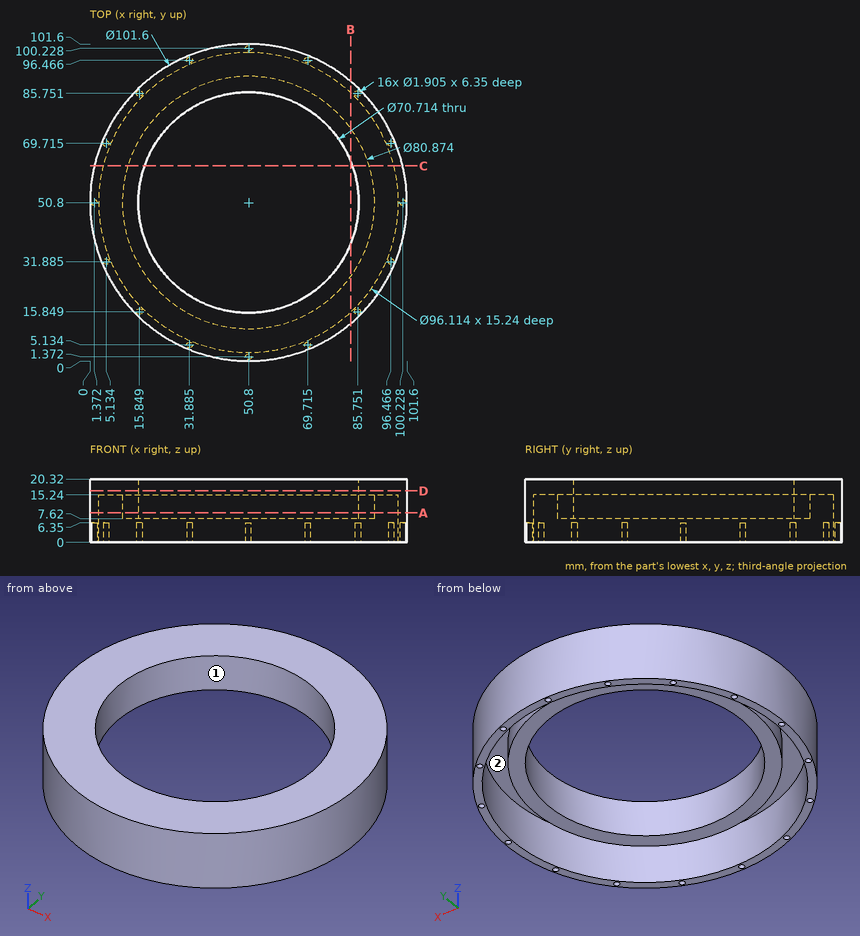
Could you check a few things on this drawing? It's one solid part, dimensions in mm from its lowest x, y, z. A direction names the side the tool comes from. Give positions to 0.01 mm unless a question says otherwise; leave off trailing zeros. Write each loop counter-clockwise with the first axis right and the second up, starting at its lowest first coordinate (ties: lowest second). Pieces come first, ordered by that corner, then holes. Notation, with made-up numbers: (89, -28) -> (93, -28) arc R10 ccw to (93, -19) -> close; hole circle Ø4 at (54, -1.75). An arc over 180 degrees is marked (long way). Answer as CSV lines item,"result". Start each with the question number.
(1) If we section it at B-B, the plane x = 83.5: Write out the boundary of the cut face in (y, z).
(2) Which directions (+Z, -Z, +X, -X, +Y, -Y) give clear straight access to the entire face, cutting with the end or side of a thin tool? Please do the marked faces 1 and 2.
(3) Please list where these lines run through material, in increasing order: line 1 (X direction, y = 50.8, z = 13.25); line 2 (X direction, y = 50.8, z = 5.75).
(4) I'm going to push flat-ended pins straight in: pin 1 Ø3 at (x, z) = (42.5, 11.5) entering from +Y; pin 2 Ø1.1 at (x, y) = (31.88, 96.47) entering from -Z; pin 3 Ø2 at (x, y) = (75, 90.5) entering from -Z. Where does each tip first touch, or does it pass through?
(5) If we section it at C-C, the plane y = 62.5: Write out the boundary of the cut face in (x, z) (1 decimal), and give its area (3 significant figures).
(6) If we section it at D-D, the plane z = 16.5: Write out the boundary of the cut face in (x, y), and give its area (3 significant figures).
(7) If we section it at A-A, the plane z = 9.5: Write out the boundary of the cut face in (x, y), and give its area (3 significant figures).
Answer list:
1,outline,"(11.92, 0) -> (15.58, 0) -> (15.58, 15.24) -> (27.01, 15.24) -> (27.01, 7.62) -> (37.35, 7.62) -> (37.35, 20.32) -> (11.92, 20.32) -> close; (64.25, 7.62) -> (74.59, 7.62) -> (74.59, 15.24) -> (86.02, 15.24) -> (86.02, 0) -> (89.68, 0) -> (89.68, 20.32) -> (64.25, 20.32) -> close"
2,face 1,"+Z, -Z"
2,face 2,"-Z"
3,line 1,"0 to 2.74, 10.36 to 15.44, 86.16 to 91.24, 98.86 to 101.6"
3,line 2,"0 to 0.42, 2.32 to 2.74, 98.86 to 99.28, 101.18 to 101.6"
4,pin 1,"y = 101.14"
4,pin 2,"z = 6.35"
4,pin 3,"z = 15.24"
5,outline,"(1.4, 0) -> (4.2, 0) -> (4.2, 15.2) -> (12.1, 15.2) -> (12.1, 7.6) -> (17.4, 7.6) -> (17.4, 20.3) -> (1.4, 20.3) -> close; (84.2, 7.6) -> (89.5, 7.6) -> (89.5, 15.2) -> (97.4, 15.2) -> (97.4, 0) -> (100.2, 0) -> (100.2, 20.3) -> (84.2, 20.3) -> close"
5,area,"331 mm^2"
6,outline,"circle Ø101.6 at (50.8, 50.8); hole circle Ø70.71 at (50.8, 50.8)"
6,area,"4,180 mm^2"
7,outline,"circle Ø101.6 at (50.8, 50.8); circle Ø80.87 at (50.8, 50.8); hole circle Ø96.11 at (50.8, 50.8); hole circle Ø70.71 at (50.8, 50.8)"
7,area,"2,060 mm^2"
